Check sheet for the modelled part. Datum: model origin and axes. Units: mm. Face numbers are marked on the shaded views. Coordinates: 2 decimals unless noted, no trailing zeros. Order: outer loops, then holes, each group sorted by start corner. A loop starts at its lowest first (then second) coordinate and runs counter-clockwise, first axis right, second up. Notation, with made-up numbers: (-39.5, 81.5) -> (-13.5, 81.5) arc R24 ccw to (-13.5, 97.5) -> close; hole circle Ø5 at (67.25, 10). An arc over 180 degrees is marked (long way). Put each result on its own line as item: value. Start each with the question number.
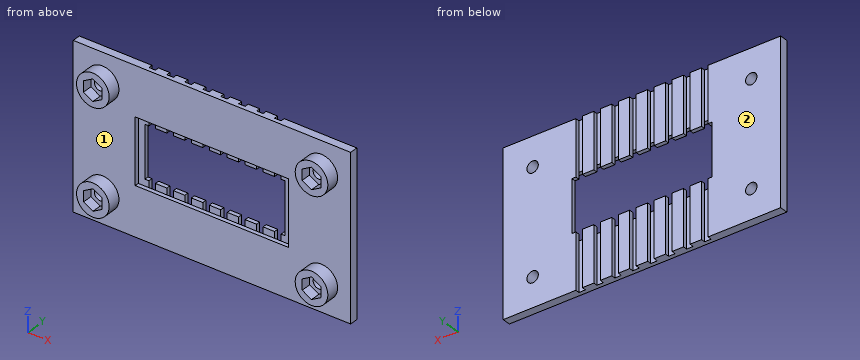
```python
from build123d import *

# Parameters (mm, degrees)
SKETCH1_W           = 85
SKETCH1_H           = 50
BASE_PLATE_DEPTH    = 2.5
SKETCH7_R           = 1.75
SCRE_CUT_DEPTH      = 5
SKETCH13_W          = 43
SKETCH13_H          = 16
CUT_EXTRUDE1_DEPTH  = 10
SKETCH15_R          = 5
BOSS_EXTRUDE3_DEPTH = 4
SKETCH18_R          = 1.75
CUT_EXTRUDE4_DEPTH  = 4
M3_NUT_DEPTH        = 3
SKETCH21_W          = 47
SKETCH21_H          = 20
SKETCH21_W_2        = 43
SKETCH21_H_2        = 16
CUT_EXTRUDE7_DEPTH  = 1.25
CUT_EXTRUDE8_REACH  = 67.744
SKETCH20_W          = 2
SKETCH20_H          = 1.25


with BuildPart() as part:
    # Sketch1 → Base Plate (new body)
    with BuildSketch(Plane(origin=(0, 0, 0), x_dir=(1, 0, 0), z_dir=(0, 1, 0))):
        Rectangle(SKETCH1_W, SKETCH1_H)
    extrude(amount=BASE_PLATE_DEPTH)

    # Sketch7 → Scre Cut (cut)
    with BuildSketch(Plane(origin=(0, 2.5, 0), x_dir=(1, 0, 0), z_dir=(0, 1, 0))):
        with Locations(Location((-33.5, 16, 0), (0, 0, 270))):
            Circle(SKETCH7_R)
        with Locations(Location((-33.5, -16, 0), (0, 0, 270))):
            Circle(SKETCH7_R)
        with Locations(Location((33.5, -16, 0), (0, 0, 270))):
            Circle(SKETCH7_R)
        with Locations(Location((33.5, 16, 0), (0, 0, 270))):
            Circle(SKETCH7_R)
    extrude(amount=-SCRE_CUT_DEPTH, mode=Mode.SUBTRACT)

    # Sketch13 → Cut-Extrude1 (cut)
    with BuildSketch(Plane(origin=(0, 2.5, 0), x_dir=(1, 0, 0), z_dir=(0, 1, 0))):
        Rectangle(SKETCH13_W, SKETCH13_H)
    extrude(amount=-CUT_EXTRUDE1_DEPTH, mode=Mode.SUBTRACT)

    # Sketch15 → Boss-Extrude3 (add)
    with BuildSketch(Plane(origin=(-42.5, 0, -25), x_dir=(1, 0, 0), z_dir=(0, -1, 0))):
        with Locations(Location((9, 9, 0), (0, 0, 90))):
            Circle(SKETCH15_R)
        with Locations(Location((9, 41, 0), (0, 0, 90))):
            Circle(SKETCH15_R)
        with Locations(Location((76, 41, 0), (0, 0, 90))):
            Circle(SKETCH15_R)
        with Locations(Location((76, 9, 0), (0, 0, 90))):
            Circle(SKETCH15_R)
    extrude(amount=BOSS_EXTRUDE3_DEPTH)

    # Sketch18 → Cut-Extrude4 (cut)
    with BuildSketch(Plane(origin=(0, 0, 0), x_dir=(1, 0, 0), z_dir=(0, 1, 0))):
        with Locations(Location((-33.5, 16, 0), (0, 0, 270))):
            Circle(SKETCH18_R)
        with Locations(Location((-33.5, -16, 0), (0, 0, 90))):
            Circle(SKETCH18_R)
        with Locations(Location((33.5, 16, 0), (0, 0, 90))):
            Circle(SKETCH18_R)
        with Locations(Location((33.5, -16, 0), (0, 0, 270))):
            Circle(SKETCH18_R)
    extrude(amount=-CUT_EXTRUDE4_DEPTH, mode=Mode.SUBTRACT)

    # Sketch19 → M3 Nut (cut)
    with BuildSketch(Plane.XZ.offset(4)):
        Polygon((-33.5, -12.709103466), (-36.35, -14.354551733), (-36.35, -17.645448267), (-33.5, -19.290896534), (-30.65, -17.645448267), (-30.65, -14.354551733), align=None)
        Polygon((-30.65, 14.354551733), (-33.5, 12.709103466), (-36.35, 14.354551733), (-36.35, 17.645448267), (-33.5, 19.290896534), (-30.65, 17.645448267), align=None)
        Polygon((30.65, -14.354551733), (33.5, -12.709103466), (36.35, -14.354551733), (36.35, -17.645448267), (33.5, -19.290896534), (30.65, -17.645448267), align=None)
        Polygon((33.5, 12.709103466), (36.35, 14.354551733), (36.35, 17.645448267), (33.5, 19.290896534), (30.65, 17.645448267), (30.65, 14.354551733), align=None)
    extrude(amount=-M3_NUT_DEPTH, mode=Mode.SUBTRACT)

    # Sketch21 → Cut-Extrude7 (cut)
    with BuildSketch(Plane.XZ):
        Rectangle(SKETCH21_W, SKETCH21_H)
        Rectangle(SKETCH21_W_2, SKETCH21_H_2, mode=Mode.SUBTRACT)
    extrude(amount=-CUT_EXTRUDE7_DEPTH, mode=Mode.SUBTRACT)

    # Cut-Extrude8: up to this face of the body (flat: up to its plane)
    cut_extrude8_end = Plane(part.part.faces().sort_by_distance((0, 1.25, 25))[0])
    # Sketch20 → Cut-Extrude8 (cut, up to the picked face)
    with BuildSketch(Plane(origin=(0, 0, -25), x_dir=(-1, 0, 0), z_dir=(0, 0, -1)), mode=Mode.PRIVATE) as cut_extrude8_sk1:
        with Locations((-2.75, 1.875)):
            Rectangle(SKETCH20_W, SKETCH20_H)
    cut_extrude8_tool1 = split(extrude(cut_extrude8_sk1.sketch, amount=-CUT_EXTRUDE8_REACH, mode=Mode.PRIVATE), bisect_by=cut_extrude8_end, keep=Keep.BOTH, mode=Mode.PRIVATE)
    # Sketch20 → Cut-Extrude8 (cut, up to the picked face)
    with BuildSketch(Plane(origin=(0, 0, -25), x_dir=(-1, 0, 0), z_dir=(0, 0, -1)), mode=Mode.PRIVATE) as cut_extrude8_sk2:
        with Locations((-8.25, 1.875)):
            Rectangle(SKETCH20_W, SKETCH20_H)
    cut_extrude8_tool2 = split(extrude(cut_extrude8_sk2.sketch, amount=-CUT_EXTRUDE8_REACH, mode=Mode.PRIVATE), bisect_by=cut_extrude8_end, keep=Keep.BOTH, mode=Mode.PRIVATE)
    # Sketch20 → Cut-Extrude8 (cut, up to the picked face)
    with BuildSketch(Plane(origin=(0, 0, -25), x_dir=(-1, 0, 0), z_dir=(0, 0, -1)), mode=Mode.PRIVATE) as cut_extrude8_sk3:
        with Locations((-13.75, 1.875)):
            Rectangle(SKETCH20_W, SKETCH20_H)
    cut_extrude8_tool3 = split(extrude(cut_extrude8_sk3.sketch, amount=-CUT_EXTRUDE8_REACH, mode=Mode.PRIVATE), bisect_by=cut_extrude8_end, keep=Keep.BOTH, mode=Mode.PRIVATE)
    # Sketch20 → Cut-Extrude8 (cut, up to the picked face)
    with BuildSketch(Plane(origin=(0, 0, -25), x_dir=(-1, 0, 0), z_dir=(0, 0, -1)), mode=Mode.PRIVATE) as cut_extrude8_sk4:
        with Locations((-19.25, 1.875)):
            Rectangle(SKETCH20_W, SKETCH20_H)
    cut_extrude8_tool4 = split(extrude(cut_extrude8_sk4.sketch, amount=-CUT_EXTRUDE8_REACH, mode=Mode.PRIVATE), bisect_by=cut_extrude8_end, keep=Keep.BOTH, mode=Mode.PRIVATE)
    # Sketch20 → Cut-Extrude8 (cut, up to the picked face)
    with BuildSketch(Plane(origin=(0, 0, -25), x_dir=(-1, 0, 0), z_dir=(0, 0, -1)), mode=Mode.PRIVATE) as cut_extrude8_sk5:
        with Locations((19.25, 1.875)):
            Rectangle(SKETCH20_W, SKETCH20_H)
    cut_extrude8_tool5 = split(extrude(cut_extrude8_sk5.sketch, amount=-CUT_EXTRUDE8_REACH, mode=Mode.PRIVATE), bisect_by=cut_extrude8_end, keep=Keep.BOTH, mode=Mode.PRIVATE)
    # Sketch20 → Cut-Extrude8 (cut, up to the picked face)
    with BuildSketch(Plane(origin=(0, 0, -25), x_dir=(-1, 0, 0), z_dir=(0, 0, -1)), mode=Mode.PRIVATE) as cut_extrude8_sk6:
        with Locations((13.75, 1.875)):
            Rectangle(SKETCH20_W, SKETCH20_H)
    cut_extrude8_tool6 = split(extrude(cut_extrude8_sk6.sketch, amount=-CUT_EXTRUDE8_REACH, mode=Mode.PRIVATE), bisect_by=cut_extrude8_end, keep=Keep.BOTH, mode=Mode.PRIVATE)
    # Sketch20 → Cut-Extrude8 (cut, up to the picked face)
    with BuildSketch(Plane(origin=(0, 0, -25), x_dir=(-1, 0, 0), z_dir=(0, 0, -1)), mode=Mode.PRIVATE) as cut_extrude8_sk7:
        with Locations((8.25, 1.875)):
            Rectangle(SKETCH20_W, SKETCH20_H)
    cut_extrude8_tool7 = split(extrude(cut_extrude8_sk7.sketch, amount=-CUT_EXTRUDE8_REACH, mode=Mode.PRIVATE), bisect_by=cut_extrude8_end, keep=Keep.BOTH, mode=Mode.PRIVATE)
    # Sketch20 → Cut-Extrude8 (cut, up to the picked face)
    with BuildSketch(Plane(origin=(0, 0, -25), x_dir=(-1, 0, 0), z_dir=(0, 0, -1)), mode=Mode.PRIVATE) as cut_extrude8_sk8:
        with Locations((2.75, 1.875)):
            Rectangle(SKETCH20_W, SKETCH20_H)
    cut_extrude8_tool8 = split(extrude(cut_extrude8_sk8.sketch, amount=-CUT_EXTRUDE8_REACH, mode=Mode.PRIVATE), bisect_by=cut_extrude8_end, keep=Keep.BOTH, mode=Mode.PRIVATE)
    add(cut_extrude8_tool1.solids().sort_by(Axis((2.75, 1.875, -25), (0, 0, 1)))[0], mode=Mode.SUBTRACT)
    add(cut_extrude8_tool2.solids().sort_by(Axis((8.25, 1.875, -25), (0, 0, 1)))[0], mode=Mode.SUBTRACT)
    add(cut_extrude8_tool3.solids().sort_by(Axis((13.75, 1.875, -25), (0, 0, 1)))[0], mode=Mode.SUBTRACT)
    add(cut_extrude8_tool4.solids().sort_by(Axis((19.25, 1.875, -25), (0, 0, 1)))[0], mode=Mode.SUBTRACT)
    add(cut_extrude8_tool5.solids().sort_by(Axis((-19.25, 1.875, -25), (0, 0, 1)))[0], mode=Mode.SUBTRACT)
    add(cut_extrude8_tool6.solids().sort_by(Axis((-13.75, 1.875, -25), (0, 0, 1)))[0], mode=Mode.SUBTRACT)
    add(cut_extrude8_tool7.solids().sort_by(Axis((-8.25, 1.875, -25), (0, 0, 1)))[0], mode=Mode.SUBTRACT)
    add(cut_extrude8_tool8.solids().sort_by(Axis((-2.75, 1.875, -25), (0, 0, 1)))[0], mode=Mode.SUBTRACT)


solid = part.part
```
1) Scan lines: line 1 along X through (y, z) = (1, -16); line 2 along X through (y, z) = (0.75, 8.5); line 3 along Z through (x, y) = (12.5, 2.25). Record each from-to range of solid material in increasing order. Write a range as [from, to].
2) Gauge pin test, flat ends, axial feed: pin 1 (1 mm diameter, centred on x = -16, z = 9, fed in from -Y); pin 2 (5.5 mm diameter, centred on x = -33.5, z = 16, fed in from -Y); pin 3 (2 mm diameter, centred on x = -7, z = -12, fed in from -Y). Record the tip position at first contact, or that the pin passes through.
3) Mould release check, pull along X, two halves, no side actions. Record for the marked faces 1 and 2: +X half, -X half, draft (parallel to the pull), parting line (faces both ways), or undercut.
4) Sectioned sample at A-A (z = -5). Record the boundary of the cut face in (x, y).
5) Sectioned sample at B-B (z = 16). State how many separate pieces and enclosed holes the cut face has, plus the area to 3 significant figures.
Entries:
1. line 1: x = [-42.5, -35.25], [-31.75, 31.75], [35.25, 42.5]
1. line 2: x = [-42.5, -23.5], [23.5, 42.5]
1. line 3: z = [-25, -8], [8, 25]
2. pin 1: stops at y = 1.25
2. pin 2: stops at y = -1
2. pin 3: stops at y = 0
3. face 1: undercut
3. face 2: draft
4. outline: (-42.5, 0) -> (-23.5, 0) -> (-23.5, 1.25) -> (-21.5, 1.25) -> (-21.5, 2.5) -> (-42.5, 2.5) -> close; (21.5, 1.25) -> (23.5, 1.25) -> (23.5, 0) -> (42.5, 0) -> (42.5, 2.5) -> (21.5, 2.5) -> close
5. separate pieces: 3
5. enclosed holes: 0
5. area: 214 mm2
